Here's how the part is built. I have some questions about the finished solid (model axes, mm). Coordinates: 2 decimals unless noted, no trailing zeros. Write each loop counter-clockwise with the first axis right and the second up, starting at its lowest first coordinate (ties: lowest second). Pieces come first, ordered by that corner, then holes.
Item 1: Please list where these lines run through material, in increasing order: line 1 (Y direction, x = 8.5, z = 460); line 2 (X direction, y = -43, z = 136.5); line 3 (X direction, y = 59.45, z = 628).
Item 2: I want a section at A-A (y = 3). Please give me the cut outline in (x, z), and give its area (3 significant figures).
Item 3: I want a section at B-B (z = -231.5). Please give me the cut outline in (x, y), and give its area (3 significant figures).
from build123d import *

# Parameters (mm, degrees)
EXTRUDE_THIN1_DEPTH      = 708
EXTRUDE_THIN1_DEPTH_BACK = 708
CUT_EXTRUDE1_REACH       = 720.724
SKETCH3_R                = 5


with BuildPart() as part:
    # Sketch2 → Extrude-Thin1 (new, two sides: drawn at the far end of the back side and taken through both)
    with BuildSketch(Plane.XY.offset(-EXTRUDE_THIN1_DEPTH_BACK)):
        with BuildLine():
            Line((-25, -60), (25, -60))
            ThreePointArc((25, -60), (28.535533906, -58.535533906), (30, -55))
            Line((30, -55), (30, 55))
            ThreePointArc((30, 55), (28.535533906, 58.535533906), (25, 60))
            Line((25, 60), (-25, 60))
            ThreePointArc((-25, 60), (-28.535533906, 58.535533906), (-30, 55))
            Line((-30, 55), (-30, -55))
            ThreePointArc((-30, -55), (-28.535533906, -58.535533906), (-25, -60))
        make_face()
        with BuildLine():
            Line((-25, -57), (25, -57))
            ThreePointArc((25, -57), (26.414213562, -56.414213562), (27, -55))
            Line((27, -55), (27, 55))
            ThreePointArc((27, 55), (26.414213562, 56.414213562), (25, 57))
            Line((25, 57), (-25, 57))
            ThreePointArc((-25, 57), (-26.414213562, 56.414213562), (-27, 55))
            Line((-27, 55), (-27, -55))
            ThreePointArc((-27, -55), (-26.414213562, -56.414213562), (-25, -57))
        make_face(mode=Mode.SUBTRACT)
    extrude(amount=EXTRUDE_THIN1_DEPTH + EXTRUDE_THIN1_DEPTH_BACK)

    # Sketch3 → Cut-Extrude1 (cut, up to next)
    with BuildSketch(Plane(origin=(0, 60, 0), x_dir=(1, 0, 0), z_dir=(0, 1, 0)), mode=Mode.PRIVATE) as cut_extrude1_sk1:
        with Locations(Location((0, 668, 0), (0, 0, 270))):
            Circle(SKETCH3_R)
    cut_extrude1_tool1 = extrude(cut_extrude1_sk1.sketch, amount=-CUT_EXTRUDE1_REACH, mode=Mode.PRIVATE) & part.part
    # Sketch3 → Cut-Extrude1 (cut, up to next)
    with BuildSketch(Plane(origin=(0, 60, 0), x_dir=(1, 0, 0), z_dir=(0, 1, 0)), mode=Mode.PRIVATE) as cut_extrude1_sk2:
        with Locations(Location((0, 628, 0), (0, 0, 270))):
            Circle(SKETCH3_R)
    cut_extrude1_tool2 = extrude(cut_extrude1_sk2.sketch, amount=-CUT_EXTRUDE1_REACH, mode=Mode.PRIVATE) & part.part
    # Sketch3 → Cut-Extrude1 (cut, up to next)
    with BuildSketch(Plane(origin=(0, 60, 0), x_dir=(1, 0, 0), z_dir=(0, 1, 0)), mode=Mode.PRIVATE) as cut_extrude1_sk3:
        with Locations(Location((0, -628, 0), (0, 0, 270))):
            Circle(SKETCH3_R)
    cut_extrude1_tool3 = extrude(cut_extrude1_sk3.sketch, amount=-CUT_EXTRUDE1_REACH, mode=Mode.PRIVATE) & part.part
    # Sketch3 → Cut-Extrude1 (cut, up to next)
    with BuildSketch(Plane(origin=(0, 60, 0), x_dir=(1, 0, 0), z_dir=(0, 1, 0)), mode=Mode.PRIVATE) as cut_extrude1_sk4:
        with Locations(Location((0, -668, 0), (0, 0, 270))):
            Circle(SKETCH3_R)
    cut_extrude1_tool4 = extrude(cut_extrude1_sk4.sketch, amount=-CUT_EXTRUDE1_REACH, mode=Mode.PRIVATE) & part.part
    add(cut_extrude1_tool1.solids().sort_by_distance((0, 60, -668))[0], mode=Mode.SUBTRACT)
    add(cut_extrude1_tool2.solids().sort_by_distance((0, 60, -628))[0], mode=Mode.SUBTRACT)
    add(cut_extrude1_tool3.solids().sort_by_distance((0, 60, 628))[0], mode=Mode.SUBTRACT)
    add(cut_extrude1_tool4.solids().sort_by_distance((0, 60, 668))[0], mode=Mode.SUBTRACT)


solid = part.part
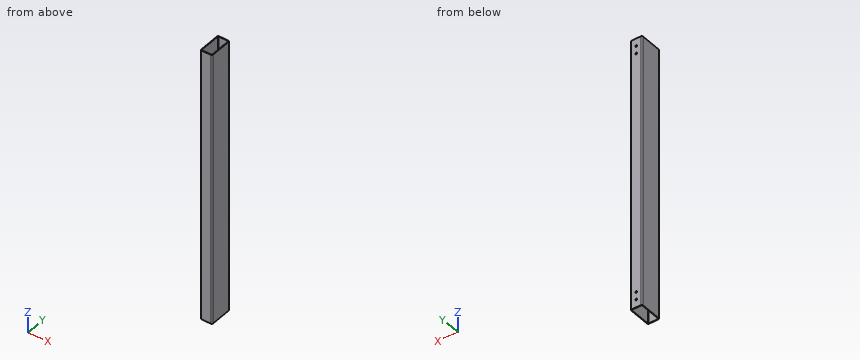
Answer:
1. line 1: y = -60 to -57, 57 to 60
1. line 2: x = -30 to -27, 27 to 30
1. line 3: x = -27.28 to -5, 5 to 27.28
2. outline: (-30, -708) - (-27, -708) - (-27, 708) - (-30, 708) - close; (27, -708) - (30, -708) - (30, 708) - (27, 708) - close
2. area: 8,500 mm2
3. outline: (-30, -55) arc R5 ccw to (-25, -60) - (25, -60) arc R5 ccw to (30, -55) - (30, 55) arc R5 ccw to (25, 60) - (-25, 60) arc R5 ccw to (-30, 55) - close; hole (-27, -55) arc R2 ccw to (-25, -57) - (25, -57) arc R2 ccw to (27, -55) - (27, 55) arc R2 ccw to (25, 57) - (-25, 57) arc R2 ccw to (-27, 55) - close
3. area: 1,030 mm2
